Input: part model. Units: mm. Frame: model coordinates. A direction names the side the tool comes from. Coordinates: 2 decimals unless noted, no trailing zeros. Loops run counter-clockwise (first coordinate to the right, second up) from the corner with the lowest first, then second, coordinate; pieces in that order, holes last. Notation, with made-up numbers: (11, 7.5) -> (38, 7.5) arc R24 cw to (38, 18.5) -> close; hole circle Ø9 at (-2, -15.75). An arc over 180 degrees is marked (long way). Put each result on its own line as item: value. Start each with the question number.
1) Pull-direction query (Y, two-part tool) for faces 1 (the flat face through (18.62, 3, 17)), 2 (the flat face through (27, -2.54, 10)), 3 (the cylindrical face through (52.616, 18.084, 9.114)); classes: pulls with the +Y half, pulls with the -Y half, needs draft (parallel to the pull), parting line crosses it, or undercut.
2) Contact query for flat-ended pins moving along their axis: P1, Ø5.5, axis at y = 1.5, z = 17, coming from the +X side; P2, Ø5, axis at x = 17.5, z = 12.5, coming from the +Y side; P3, Ø10, axis at x = 6.5, y = 9.5, coming from the +Z side. Output: stop coordinate, or through.
3) Cut plane C-C (y = 0.75). Return the cut outline in (x, z) (3 decimals), plus the area to 3 significant figures.
4) Cut plane B-B (y = 6.75). Return the cut outline in (x, z) (3 decimals).
5) Material intervals for L1, parallel to X at y = 3, z = 10 (3 decimals); L2, parallel to Z at x = 13, y = 8 (3 decimals); L3, parallel to X at y = 5, z = 14, sorted ascending.
6) Set-up query: faces 4 (the flat face through (28, 0, 10)), 5 (the cylindrical face through (55.405, 17.99, 9.427)), 6 (the flat face through (52.07, 8, 9)), 7 (the flat face through (26, 5.46, 17)). Return all of +Z, -Z, +X, -X, +Y, -Y with unobstructed straight access to the full face (end or side cutting, diameter ignored); none if empty.
from build123d import *

# Parameters (mm, degrees)
F0_W         = 19.05
F0_H         = 19.05
F1_DEPTH     = 55.88
F2_W         = 47.625
F2_H         = 9.525
F3_DEPTH     = 25.4
F4_W         = 55.7279027998
F4_H         = 19.3847697228
F5_DEPTH     = 2.54
F6_T1_DEPTH  = 50.8
F6_T3_DEPTH  = 13.97
F6_T5_DEPTH  = 47.625
F6_T7_DEPTH  = 9.525
F6_T9_DEPTH  = 16.51
F6_T11_DEPTH = 25.4
F6_T13_DEPTH = 22.86
F6_S17_W     = 2.5908
F6_S17_H     = 2.5908
F6_T18_DEPTH = 2.5908
F6_S23_W     = 2.5908
F6_S23_H     = 2.5908
F6_T24_DEPTH = 2.5908
F6_S29_W     = 2.5908
F6_S29_H     = 2.5908
F6_T30_DEPTH = 2.5908
F6_S35_W     = 2.5908
F6_S35_H     = 2.5908
F6_T36_DEPTH = 2.5908
F6_T43_DEPTH = 53.975
F6_T48_DEPTH = 15.875
F6_T56_DEPTH = 53.975
F6_T61_DEPTH = 15.875
F6_T69_DEPTH = 15.875
F6_T74_DEPTH = 53.975
F6_T82_DEPTH = 53.975
F6_T87_DEPTH = 15.875
F7_W         = 15.8100910485
F7_H         = 5.4600955918
F8_DEPTH     = 12.7


# Not quite as in the source:
# - a fillet or chamfer that OpenCascade refuses, or shapes differently, is made with other operations: its cross-section is extruded or revolved along the edge and cut away or added


with BuildPart() as f1:
    # F0 (on Right) → F1 (new body)
    with BuildSketch(Plane.YZ):
        with Locations((9.525, 9.525)):
            Rectangle(F0_W, F0_H)
    extrude(amount=F1_DEPTH)

    # F2 (on face) → F3 (cut)
    with BuildSketch(Plane.XZ):
        with Locations((28.2575, 9.2075)):
            Rectangle(F2_W, F2_H)
    extrude(amount=-F3_DEPTH, mode=Mode.SUBTRACT)

    # F4 (on Front) → F5 (join)
    with BuildSketch(Plane.XZ):
        with Locations((27.8639513999, 9.6923848614)):
            Rectangle(F4_W, F4_H)
    extrude(amount=F5_DEPTH)

    # F6: fillet of radius 2.54 on 12 edges, made by hand

    # F6_s2 → F6_t1 (cut)
    with BuildSketch(Plane.YZ.offset(2.54)):
        with BuildLine():
            ThreePointArc((19.05, 2.54), (18.3060512242, 0.7439487758), (16.51, 0))
            Line((16.51, 0), (19.05, 0))
            Line((19.05, 0), (19.05, 2.54))
        make_face()
        with BuildLine():
            ThreePointArc((16.51, 19.05), (18.3060512242, 18.3060512242), (19.05, 16.51))
            Line((19.05, 16.51), (19.05, 19.05))
            Line((19.05, 19.05), (16.51, 19.05))
        make_face()
    extrude(amount=F6_T1_DEPTH, mode=Mode.SUBTRACT)

    # F6_s4 → F6_t3 (cut)
    with BuildSketch(Plane.XY.offset(2.54)):
        with BuildLine():
            ThreePointArc((0, 16.51), (0.7439487758, 18.3060512242), (2.54, 19.05))
            Line((2.54, 19.05), (0, 19.05))
            Line((0, 19.05), (0, 16.51))
        make_face()
        with BuildLine():
            ThreePointArc((53.34, 19.05), (55.1360512242, 18.3060512242), (55.88, 16.51))
            Line((55.88, 16.51), (55.88, 19.05))
            Line((55.88, 19.05), (53.34, 19.05))
        make_face()
    extrude(amount=F6_T3_DEPTH, mode=Mode.SUBTRACT)

    # F6_s6 → F6_t5 (cut)
    with BuildSketch(Plane.YZ.offset(4.445)):
        with BuildLine():
            ThreePointArc((19.05, 16.51), (18.3060512242, 14.7139487758), (16.51, 13.97))
            Line((16.51, 13.97), (19.05, 13.97))
            Line((19.05, 13.97), (19.05, 16.51))
        make_face()
        with BuildLine():
            ThreePointArc((19.05, 1.905), (18.3060512242, 3.7010512242), (16.51, 4.445))
            Line((16.51, 4.445), (19.05, 4.445))
            Line((19.05, 4.445), (19.05, 1.905))
        make_face()
    extrude(amount=F6_T5_DEPTH, mode=Mode.SUBTRACT)

    # F6_s8 → F6_t7 (cut)
    with BuildSketch(Plane.XY.offset(4.445)):
        with BuildLine():
            ThreePointArc((1.905, 19.05), (3.7010512242, 18.3060512242), (4.445, 16.51))
            Line((4.445, 16.51), (4.445, 19.05))
            Line((4.445, 19.05), (1.905, 19.05))
        make_face()
        with BuildLine():
            ThreePointArc((54.61, 19.05), (52.8139487758, 18.3060512242), (52.07, 16.51))
            Line((52.07, 16.51), (52.07, 19.05))
            Line((52.07, 19.05), (54.61, 19.05))
        make_face()
    extrude(amount=F6_T7_DEPTH, mode=Mode.SUBTRACT)

    # F6_s10 → F6_t9 (cut)
    with BuildSketch(Plane.XZ.offset(-16.51)):
        with BuildLine():
            ThreePointArc((2.54, 19.05), (0.7439487758, 18.3060512242), (0, 16.51))
            Line((0, 16.51), (0, 19.05))
            Line((0, 19.05), (2.54, 19.05))
        make_face()
        with BuildLine():
            ThreePointArc((53.34, 19.05), (55.1360512242, 18.3060512242), (55.88, 16.51))
            Line((55.88, 16.51), (55.88, 19.05))
            Line((55.88, 19.05), (53.34, 19.05))
        make_face()
    extrude(amount=F6_T9_DEPTH, mode=Mode.SUBTRACT)

    # F6_s12 → F6_t11 (cut)
    with BuildSketch(Plane.XZ.offset(-16.51)):
        with BuildLine():
            ThreePointArc((0, 2.54), (0.7439487758, 0.7439487758), (2.54, 0))
            Line((2.54, 0), (0, 0))
            Line((0, 0), (0, 2.54))
        make_face()
    extrude(amount=F6_T11_DEPTH, mode=Mode.SUBTRACT)

    # F6_s14 → F6_t13 (cut)
    with BuildSketch(Plane.XZ.offset(-16.51)):
        with BuildLine():
            ThreePointArc((55.88, 2.54), (55.1360512242, 0.7439487758), (53.34, 0))
            Line((53.34, 0), (55.88, 0))
            Line((55.88, 0), (55.88, 2.54))
        make_face()
    extrude(amount=F6_T13_DEPTH, mode=Mode.SUBTRACT)


with BuildPart() as f6_tool16:
    # F6_s17 → F6_t18 (new body)
    with BuildSketch(Plane.YZ.offset(2.54)):
        with Locations((17.8054, 1.2446)):
            Rectangle(F6_S17_W, F6_S17_H)
    extrude(amount=-F6_T18_DEPTH)

    # F6_s19 → F6_t20 (revolve, cut)
    with BuildSketch(Plane(origin=(2.54, 16.51, 2.54), x_dir=(0, -0.7071067812, 0.7071067812), z_dir=(0, -0.7071067812, -0.7071067812))):
        with BuildLine():
            ThreePointArc((0, -2.54), (2.54, 0), (0, 2.54))
            Line((0, 2.54), (0, -2.54))
        make_face()
    revolve(axis=Axis((2.54, 16.51, 2.54), (-1, 0, 0)), mode=Mode.SUBTRACT)


with BuildPart() as f1_1:
    add(f1.part)

    # F6_t15: cut F6_tool16
    add(f6_tool16.part, mode=Mode.SUBTRACT)


with BuildPart() as f6_tool22:
    # F6_s23 → F6_t24 (new body)
    with BuildSketch(Plane.YZ.offset(53.34)):
        with Locations((17.8054, 1.2446)):
            Rectangle(F6_S23_W, F6_S23_H)
    extrude(amount=F6_T24_DEPTH)

    # F6_s25 → F6_t26 (revolve, cut)
    with BuildSketch(Plane(origin=(53.34, 16.51, 2.54), x_dir=(0, -0.7071067812, 0.7071067812), z_dir=(0, 0.7071067812, 0.7071067812))):
        with BuildLine():
            ThreePointArc((0, -2.54), (2.54, 0), (0, 2.54))
            Line((0, 2.54), (0, -2.54))
        make_face()
    revolve(axis=Axis((53.34, 16.51, 2.54), (1, 0, 0)), mode=Mode.SUBTRACT)


with BuildPart() as f1_2:
    add(f1_1.part)

    # F6_t21: cut F6_tool22
    add(f6_tool22.part, mode=Mode.SUBTRACT)


with BuildPart() as f6_tool28:
    # F6_s29 → F6_t30 (new body)
    with BuildSketch(Plane.XY.offset(16.51)):
        with Locations((1.2446, 17.8054)):
            Rectangle(F6_S29_W, F6_S29_H)
    extrude(amount=F6_T30_DEPTH)

    # F6_s31 → F6_t32 (revolve, cut)
    with BuildSketch(Plane(origin=(2.54, 16.51, 16.51), x_dir=(0.7071067812, -0.7071067812, 0), z_dir=(-0.7071067812, -0.7071067812, 0))):
        with BuildLine():
            ThreePointArc((0, -2.54), (2.54, 0), (0, 2.54))
            Line((0, 2.54), (0, -2.54))
        make_face()
    revolve(axis=Axis((2.54, 16.51, 16.51), (0, 0, 1)), mode=Mode.SUBTRACT)


with BuildPart() as f1_3:
    add(f1_2.part)

    # F6_t27: cut F6_tool28
    add(f6_tool28.part, mode=Mode.SUBTRACT)


with BuildPart() as f6_tool34:
    # F6_s35 → F6_t36 (new body)
    with BuildSketch(Plane.XY.offset(16.51)):
        with Locations((54.6354, 17.8054)):
            Rectangle(F6_S35_W, F6_S35_H)
    extrude(amount=F6_T36_DEPTH)

    # F6_s37 → F6_t38 (revolve, cut)
    with BuildSketch(Plane(origin=(53.34, 16.51, 16.51), x_dir=(-0.7071067812, -0.7071067812, 0), z_dir=(-0.7071067812, 0.7071067812, 0))):
        with BuildLine():
            ThreePointArc((0, -2.54), (2.54, 0), (0, 2.54))
            Line((0, 2.54), (0, -2.54))
        make_face()
    revolve(axis=Axis((53.34, 16.51, 16.51), (0, 0, 1)), mode=Mode.SUBTRACT)


with BuildPart() as f1_4:
    add(f1_3.part)

    # F6_t33: cut F6_tool34
    add(f6_tool34.part, mode=Mode.SUBTRACT)


with BuildPart() as f6_tool41:
    # F6_s42 → F6_t43 (new body)
    with BuildSketch(Plane.YZ.offset(58.42)):
        with BuildLine():
            ThreePointArc((19.05, 16.51), (18.3060512242, 14.7139487758), (16.51, 13.97))
            Line((16.51, 13.97), (19.05, 13.97))
            Line((19.05, 13.97), (19.05, 16.51))
        make_face()
    extrude(amount=-F6_T43_DEPTH)

    split(bisect_by=Plane.YZ.offset(52.07), keep=Keep.TOP)

    split(bisect_by=Plane.YZ.offset(55.88), keep=Keep.BOTTOM)


with BuildPart() as f6_tool46:
    # F6_s47 → F6_t48 (new body)
    with BuildSketch(Plane.XY.offset(4.445)):
        with BuildLine():
            ThreePointArc((54.61, 19.05), (52.8139487758, 18.3060512242), (52.07, 16.51))
            Line((52.07, 16.51), (52.07, 19.05))
            Line((52.07, 19.05), (54.61, 19.05))
        make_face()
    extrude(amount=F6_T48_DEPTH)

    split(bisect_by=Plane.XY.offset(19.05), keep=Keep.BOTTOM)

    split(bisect_by=Plane.XY.offset(13.97), keep=Keep.TOP)


with BuildPart() as f6_tool41_1:
    add(f6_tool41.part)

    # F6_t51: intersect F6_tool46
    add(f6_tool46.part, mode=Mode.INTERSECT)


with BuildPart() as f1_5:
    add(f1_4.part)

    # F6_t39: cut F6_tool41
    add(f6_tool41_1.part, mode=Mode.SUBTRACT)


with BuildPart() as f6_tool54:
    # F6_s55 → F6_t56 (new body)
    with BuildSketch(Plane.YZ.offset(52.07)):
        with BuildLine():
            ThreePointArc((19.05, 16.51), (18.3060512242, 14.7139487758), (16.51, 13.97))
            Line((16.51, 13.97), (19.05, 13.97))
            Line((19.05, 13.97), (19.05, 16.51))
        make_face()
    extrude(amount=-F6_T56_DEPTH)

    split(bisect_by=Plane.YZ, keep=Keep.TOP)

    split(bisect_by=Plane.YZ.offset(4.445), keep=Keep.BOTTOM)


with BuildPart() as f6_tool59:
    # F6_s60 → F6_t61 (new body)
    with BuildSketch(Plane.XY.offset(20.32)):
        with BuildLine():
            ThreePointArc((1.905, 19.05), (3.7010512242, 18.3060512242), (4.445, 16.51))
            Line((4.445, 16.51), (4.445, 19.05))
            Line((4.445, 19.05), (1.905, 19.05))
        make_face()
    extrude(amount=-F6_T61_DEPTH)

    split(bisect_by=Plane.XY.offset(19.05), keep=Keep.BOTTOM)

    split(bisect_by=Plane.XY.offset(13.97), keep=Keep.TOP)


with BuildPart() as f6_tool54_1:
    add(f6_tool54.part)

    # F6_t64: intersect F6_tool59
    add(f6_tool59.part, mode=Mode.INTERSECT)


with BuildPart() as f1_6:
    add(f1_5.part)

    # F6_t52: cut F6_tool54
    add(f6_tool54_1.part, mode=Mode.SUBTRACT)


with BuildPart() as f6_tool67:
    # F6_s68 → F6_t69 (new body)
    with BuildSketch(Plane.XY.offset(13.97)):
        with BuildLine():
            ThreePointArc((1.905, 19.05), (3.7010512242, 18.3060512242), (4.445, 16.51))
            Line((4.445, 16.51), (4.445, 19.05))
            Line((4.445, 19.05), (1.905, 19.05))
        make_face()
    extrude(amount=-F6_T69_DEPTH)

    split(bisect_by=Plane.XY.offset(4.445), keep=Keep.BOTTOM)

    split(bisect_by=Plane.XY, keep=Keep.TOP)


with BuildPart() as f6_tool72:
    # F6_s73 → F6_t74 (new body)
    with BuildSketch(Plane.YZ.offset(-1.905)):
        with BuildLine():
            ThreePointArc((19.05, 1.905), (18.3060512242, 3.7010512242), (16.51, 4.445))
            Line((16.51, 4.445), (19.05, 4.445))
            Line((19.05, 4.445), (19.05, 1.905))
        make_face()
    extrude(amount=F6_T74_DEPTH)

    split(bisect_by=Plane.YZ, keep=Keep.TOP)

    split(bisect_by=Plane.YZ.offset(4.445), keep=Keep.BOTTOM)


with BuildPart() as f6_tool67_1:
    add(f6_tool67.part)

    # F6_t77: intersect F6_tool72
    add(f6_tool72.part, mode=Mode.INTERSECT)


with BuildPart() as f1_7:
    add(f1_6.part)

    # F6_t65: cut F6_tool67
    add(f6_tool67_1.part, mode=Mode.SUBTRACT)


with BuildPart() as f6_tool80:
    # F6_s81 → F6_t82 (new body)
    with BuildSketch(Plane.YZ.offset(4.445)):
        with BuildLine():
            ThreePointArc((19.05, 1.905), (18.3060512242, 3.7010512242), (16.51, 4.445))
            Line((16.51, 4.445), (19.05, 4.445))
            Line((19.05, 4.445), (19.05, 1.905))
        make_face()
    extrude(amount=F6_T82_DEPTH)

    split(bisect_by=Plane.YZ.offset(52.07), keep=Keep.TOP)

    split(bisect_by=Plane.YZ.offset(55.88), keep=Keep.BOTTOM)


with BuildPart() as f6_tool85:
    # F6_s86 → F6_t87 (new body)
    with BuildSketch(Plane.XY.offset(-1.905)):
        with BuildLine():
            ThreePointArc((54.61, 19.05), (52.8139487758, 18.3060512242), (52.07, 16.51))
            Line((52.07, 16.51), (52.07, 19.05))
            Line((52.07, 19.05), (54.61, 19.05))
        make_face()
    extrude(amount=F6_T87_DEPTH)

    split(bisect_by=Plane.XY.offset(4.445), keep=Keep.BOTTOM)

    split(bisect_by=Plane.XY, keep=Keep.TOP)


with BuildPart() as f6_tool80_1:
    add(f6_tool80.part)

    # F6_t90: intersect F6_tool85
    add(f6_tool85.part, mode=Mode.INTERSECT)


with BuildPart() as f1_8:
    add(f1_7.part)

    # F6_t78: cut F6_tool80
    add(f6_tool80_1.part, mode=Mode.SUBTRACT)

    # F7 (on face) → F8 (cut)
    with BuildSketch(Plane.XY.offset(19.05)):
        with Locations((26.5251491219, 2.7300477959)):
            Rectangle(F7_W, F7_H)
    extrude(amount=-F8_DEPTH, mode=Mode.SUBTRACT)


solid = f1_8.part
Results found:
1. face 1: undercut
1. face 2: pulls with the -Y half
1. face 3: pulls with the +Y half
2. P1: stops at x = 55.88
2. P2: stops at y = 18.55
2. P3: stops at z = 19.05
3. outline: (0, 2.54) arc R2.54 ccw to (2.54, 0) -> (53.34, 0) arc R2.54 ccw to (55.88, 2.54) -> (55.88, 16.51) arc R2.54 ccw to (53.34, 19.05) -> (34.43, 19.05) -> (34.43, 13.97) -> (52.07, 13.97) -> (52.07, 4.445) -> (4.445, 4.445) -> (4.445, 13.97) -> (18.62, 13.97) -> (18.62, 19.05) -> (2.54, 19.05) arc R2.54 ccw to (0, 16.51) -> close
3. area: 525 mm2
4. outline: (0, 2.54) arc R2.54 ccw to (2.54, 0) -> (53.34, 0) arc R2.54 ccw to (55.88, 2.54) -> (55.88, 16.51) arc R2.54 ccw to (53.34, 19.05) -> (2.54, 19.05) arc R2.54 ccw to (0, 16.51) -> close; hole (4.445, 4.445) -> (52.07, 4.445) -> (52.07, 13.97) -> (4.445, 13.97) -> close
5. L1: x = 0 to 4.445, 52.07 to 55.88
5. L2: z = 0 to 4.445, 13.97 to 19.05
5. L3: x = 0 to 18.62, 34.43 to 55.88
6. face 4: none
6. face 5: +Z, -Z, +X, +Y
6. face 6: +Y
6. face 7: +Z
